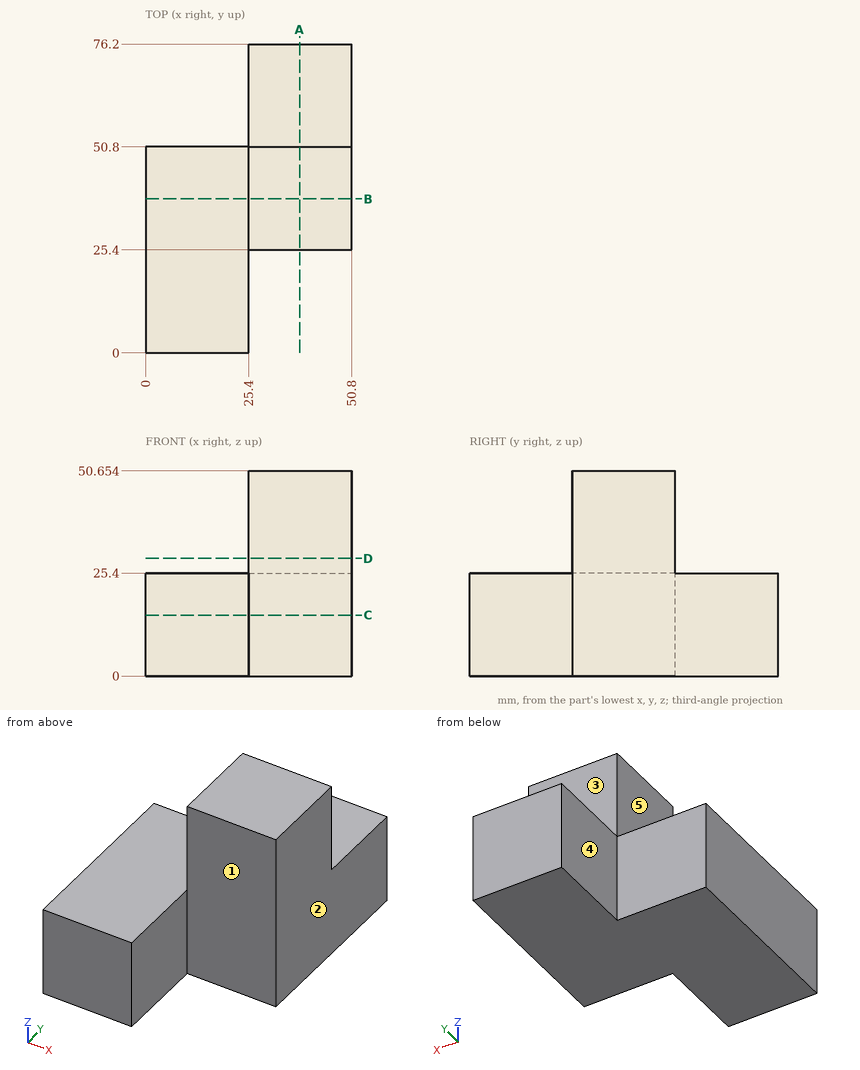
Check sheet for the drawn part. Datum: minimum x, y, z corner. Units: mm. A direction names the side the tool comes from. Give positions to 0.01 mm unless a question says otherwise; leave off trailing zeros. Loops run counter-clockwise (first coordinate to the right, second up) from the corner with the lowest first, then second, coordinate; pieces in that order, holes last. Notation, with made-up numbers: M 82.5,-33 L 125.5,-33 A15 ccw 125.5,-4 Z; hole C 53,11 d8. An arc over 180 degrees is marked long. Return JSON: item names as keys, results as strings.
1) Gauge pin test, flat ends, axial feed: P1, Ø7.5, axis at x = 32.5, y = 57.5, coming from the +Z side; P2, Ø7.5, axis at y = 37, z = 33.5, coming from the -X side; P3, Ø1, axis at x = 44.5, z = 44.5, coming from the -Y side. Record the tip position at first contact, or that the pin passes through.
Findings:
{"P1": "stops at z = 25.4", "P2": "stops at x = 25.4", "P3": "stops at y = 25.4"}
2) Section check D-D, the plane z = 29. Enter the section's corners in (x, y).
Findings:
{"outline": "M 25.4,25.4 L 50.8,25.4 L 50.8,50.8 L 25.4,50.8 Z"}
3) Tool access check on the marked faces 1, 2, 3, 4 and 5. Record the directions out of +Z, -Z, +X, -X, +Y, -Y that give a thin tool (end or side, any length) a straight path to the whole face; none if there is none.
Findings:
{"face 1": "+Z, -Z, +X, -Y", "face 2": "+Z, -Z, +X, +Y, -Y", "face 3": "+Z, +X, -X, +Y", "face 4": "+Z, -Z, -X, +Y", "face 5": "+Z, -X, +Y, -Y"}
4) Section check C-C, the plane z = 15. Enter the section's corners in (x, y), and give its area (3 significant figures).
Findings:
{"outline": "M 0,0 L 25.4,0 L 25.4,25.4 L 50.8,25.4 L 50.8,76.2 L 25.4,76.2 L 25.4,50.8 L 0,50.8 Z", "area": "2,580 mm2"}
5) Section check A-A, the plane x = 38. Enter the section's corners in (y, z), and give its area (3 significant figures).
Findings:
{"outline": "M 25.4,0 L 76.2,0 L 76.2,25.4 L 50.8,25.4 L 50.8,50.65 L 25.4,50.65 Z", "area": "1,930 mm2"}
6) Section check B-B, the plane y = 38. Enter the section's corners in (x, z).
Findings:
{"outline": "M 0,0 L 50.8,0 L 50.8,50.65 L 25.4,50.65 L 25.4,25.4 L 0,25.4 Z"}
7) Material ranges on L1, parallel to Y at x = 30, z = 46.5; L2, parallel to Y at x = 42.5, z = 7.5; L3, parallel to Z at x = 13, y = 37.5, recorded low to high. Write a range as [from, to].
Findings:
{"L1": "y = [25.4, 50.8]", "L2": "y = [25.4, 76.2]", "L3": "z = [0, 25.4]"}
